from build123d import *

# Parameters (mm, degrees)
BOSS_EXTRUDE1_DEPTH = 6.35
CUT_EXTRUDE1_REACH  = 8.35
SKETCH2_R           = 1.63195


with BuildPart() as part:
    # Sketch1 → Boss-Extrude1 (new body)
    with BuildSketch(Plane(origin=(0, 0, 0), x_dir=(0, 1, 0), z_dir=(0, 0, 1))):
        with BuildLine():
            Line((-9.525, 16.497783942), (-6.35, 10.998522628))
            ThreePointArc((-6.35, 10.998522628), (0, 12.7), (6.35, 10.998522628))
            Line((6.35, 10.998522628), (9.525, 16.497783942))
            ThreePointArc((9.525, 16.497783942), (0, 19.05), (-9.525, 16.497783942))
        make_face()
    extrude(amount=BOSS_EXTRUDE1_DEPTH)

    # Sketch2 → Cut-Extrude1 (cut, up to next)
    with BuildSketch(Plane.XY.offset(6.35), mode=Mode.PRIVATE) as cut_extrude1_sk1:
        with Locations((-15.057884182, 5.027499276)):
            Circle(SKETCH2_R)
    cut_extrude1_tool1 = extrude(cut_extrude1_sk1.sketch, amount=-CUT_EXTRUDE1_REACH, mode=Mode.PRIVATE) & part.part
    add(cut_extrude1_tool1.solids().sort_by_distance((-15.057884, 5.027499, 6.35))[0], mode=Mode.SUBTRACT)
    # Sketch2 → Cut-Extrude1 (cut, up to next)
    with BuildSketch(Plane.XY.offset(6.35), mode=Mode.PRIVATE) as cut_extrude1_sk2:
        with Locations((-15.057884182, -5.027499276)):
            Circle(SKETCH2_R)
    cut_extrude1_tool2 = extrude(cut_extrude1_sk2.sketch, amount=-CUT_EXTRUDE1_REACH, mode=Mode.PRIVATE) & part.part
    add(cut_extrude1_tool2.solids().sort_by_distance((-15.057884, -5.027499, 6.35))[0], mode=Mode.SUBTRACT)


solid = part.part
The listing builds one solid part. Answer for the finished solid, in the listing's coordinates (mm). Coordinates: 2 decimals unless noted, no trailing zeros. Write each loop counter-clockwise with the first axis right and the second up, starting at its lowest first coordinate (ties: lowest second). Pieces come first, ordered by that corner, then holes. Notation, with made-up numbers: (86, 6) - (110, 6) arc R17 cw to (110, 17) - close; hole circle Ø2 at (22.5, 21). An arc over 180 degrees is marked (long way). Answer as CSV lines item,"result".
1. Find section C-C (z = 2.25). Give the number of separate pieces and of enclosed holes in the cut face, plus the area to 3 significant figures.
Computed values:
separate pieces,"1"
enclosed holes,"2"
area,"88.8 mm²"
2. Find section D-D (x = -15.5). Give the vertices of the cut face in (y, z).
Computed values:
outline,"(-8.95, 0) - (-6.6, 0) - (-6.6, 6.35) - (-8.95, 6.35) - close; (-3.46, 0) - (3.46, 0) - (3.46, 6.35) - (-3.46, 6.35) - close; (6.6, 0) - (8.95, 0) - (8.95, 6.35) - (6.6, 6.35) - close"
3. Find section B-B (y = 4.25). Give the vertices of the cut face in (x, z).
Computed values:
outline,"(-18.57, 0) - (-16.49, 0) - (-16.49, 6.35) - (-18.57, 6.35) - close; (-13.62, 0) - (-11.97, 0) - (-11.97, 6.35) - (-13.62, 6.35) - close"
4. Given P1, Ø2, axis at x = -18, y = 7.5, coming from the -Z side; P2, Ø1, axis at y = -5, z = 3, coming from the -X side, each flat-ended and moving along its own axis, determine where each tip first touches the part or whether it passes through.
Computed values:
P1,"stops at z = 0"
P2,"stops at x = -18.51"
5. Find section A-A (x = -14.5). Give the vertices of the cut face in (y, z).
Computed values:
outline,"(-8.37, 0) - (-6.56, 0) - (-6.56, 6.35) - (-8.37, 6.35) - close; (-3.49, 0) - (3.49, 0) - (3.49, 6.35) - (-3.49, 6.35) - close; (6.56, 0) - (8.37, 0) - (8.37, 6.35) - (6.56, 6.35) - close"
6. Straight lines are drawn through the part: line 1 (Y direction, x = -15, z = 3); line 2 (Y direction, x = -15.75, z = 1); line 3 (X direction, y = 5, z = 5.75). For each, find the intervals that lie inside material, in ascending order. Write a range as [from, to].
Computed values:
line 1,"y = [-8.66, -6.66], [-3.4, 3.4], [6.66, 8.66]"
line 2,"y = [-9.09, -6.51], [-3.55, 3.55], [6.51, 9.09]"
line 3,"x = [-18.38, -16.69], [-13.43, -11.67]"
7. Determine the mould class of faces 1 (the flat face through (-13.71, 7.915, 3.131)), 2 (the cylindrical face through (-16.69, 5.1, 3.22)), 3 (the cylindrical face through (-19.05, 0.14, 3.13)) for opening direction Y: +Y half, -Y half, draft (parallel to the pull), parting line (faces both ways), or undercut.
Computed values:
face 1,"+Y half"
face 2,"undercut"
face 3,"parting line"
